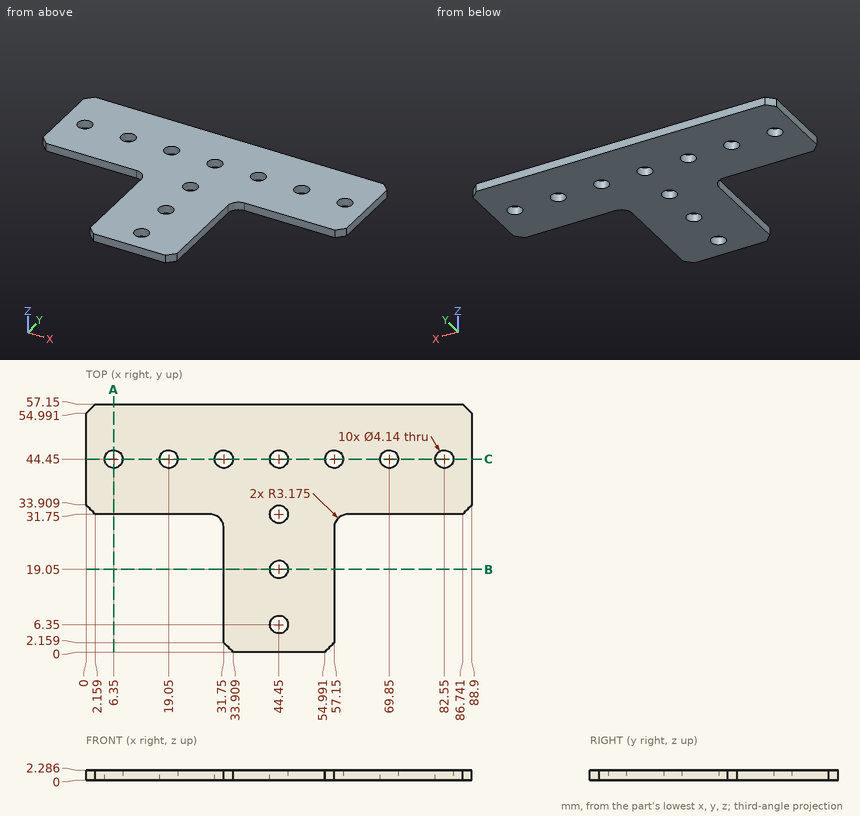
Design review of the part shown in the three views and the two pictorial views. Dimensions are in mm from the part's minimum x, y and z. Coordinates: 2 decimals unless noted, no trailing zeros. Loops run counter-clockwise (first coordinate to the right, second up) from the corner with the lowest first, then second, coordinate; pieces in that order, holes last. Notation, with made-up numbers: M -1,60.5 L 23,60.5 A18 ccw 23,86.5 Z; hole C 50.5,26 d10. An arc over 180 degrees is marked long. Put each result on its own line as item: value. Start each with the question number.
Q1. Clearance check with flat-ended pins moving along their axes: pin 1 (6.5 mm diameter, centred on x = 6.35, y = 44.45, fed in from +Z); pin 2 (4 mm diameter, centred on x = 29.5, y = 25.5, fed in from -Z); pin 3 (1 mm diameter, centred on x = 25.5, z = 1.5, fed in from -Y); pin 4 (1.1 mm diameter, centred on y = 15.5, z = 1, fed in from -X). State where each tip first meets the part, or that it passes through.
Q2. Wall thickness on line 1 (Y direction, x = 44.45, z = 1.1); line 2 (Y direction, x = 82.5, z = 0.45); line 3 (Y direction, x = 46, z = 2.2): over which ranges is each line inside the solid? List them lowest first.
Q3. Add section A-A (x = 6.35). Write out the cut boundary in (y, z).
Q4. Add section C-C (y = 44.45). Count the separate pieces of the cut face and the enclosed holes in it, and give its area (3 significant figures).
Answers:
1. pin 1: stops at z = 2.29
1. pin 2: passes through
1. pin 3: stops at y = 31.75
1. pin 4: stops at x = 31.75
2. line 1: y = 0 to 4.28, 8.42 to 16.98, 21.12 to 29.68, 33.82 to 42.38, 46.52 to 57.15
2. line 2: y = 31.75 to 42.38, 46.52 to 57.15
2. line 3: y = 0 to 4.98, 7.72 to 17.68, 20.42 to 30.38, 33.12 to 43.08, 45.82 to 57.15
3. outline: M 31.75,0 L 42.38,0 L 42.38,2.29 L 31.75,2.29 Z; M 46.52,0 L 57.15,0 L 57.15,2.29 L 46.52,2.29 Z
4. separate pieces: 8
4. enclosed holes: 0
4. area: 137 mm^2
